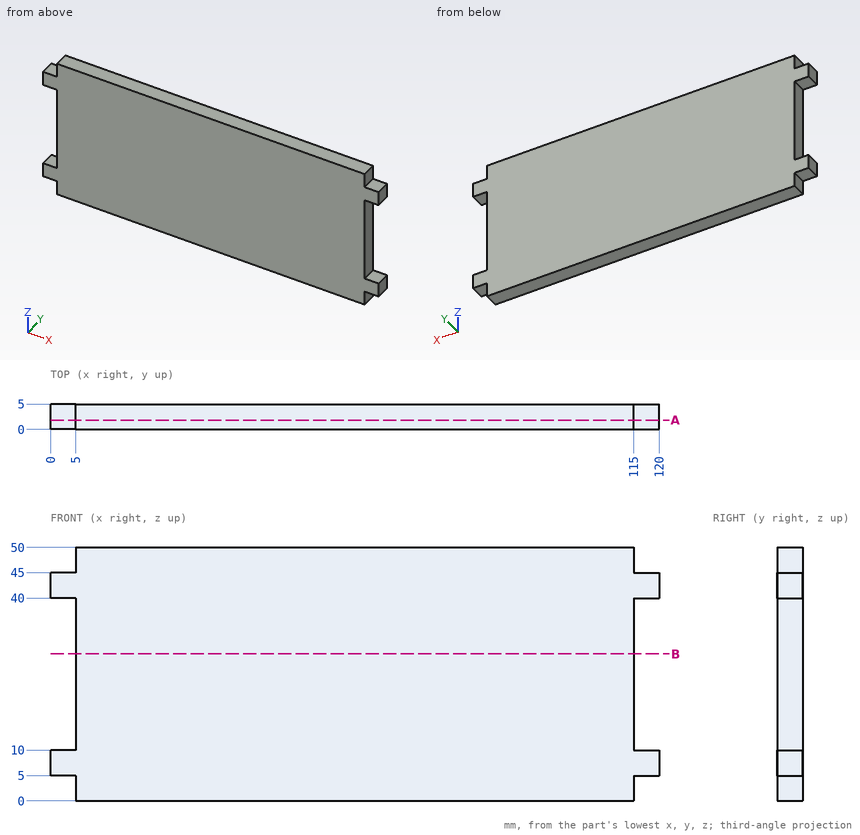
The drawing under review shows one solid part. Ordinate dimensions are in mm from its lowest x, y, z. Coordinates: 2 decimals unless noted, no trailing zeros. Loops run counter-clockwise (first coordinate to the right, second up) from the corner with the lowest first, then second, coordinate; pieces in that order, holes last.
Item 1: Clearance check with flat-ended pins moving along their axes: pin 1 (2.5 mm diameter, centred on x = 2.5, y = 3.5, fed in from -Z); pin 2 (2.5 mm diameter, centred on y = 3, z = 19.5, fed in from +X); pin 3 (2.5 mm diameter, centred on y = 1.5, z = 46.5, fed in from -X). State where each tip first meets the part, or that it passes through.
Completed:
pin 1: stops at z = 5
pin 2: stops at x = 115
pin 3: stops at x = 5
Item 2: Add section A-A (y = 1.8). Write out the cut boundary in (x, z).
Completed:
outline: (0, 5) - (5, 5) - (5, 0) - (115, 0) - (115, 5) - (120, 5) - (120, 10) - (115, 10) - (115, 40) - (120, 40) - (120, 45) - (115, 45) - (115, 50) - (5, 50) - (5, 45) - (0, 45) - (0, 40) - (5, 40) - (5, 10) - (0, 10) - close
Item 3: Add section B-B (z = 29). Write out the cut boundary in (x, y).
Completed:
outline: (5, 0) - (115, 0) - (115, 5) - (5, 5) - close
Item 4: Wall thickness on L1, parallel to X at y = 3.1, z = 12.5: over which ranges is the line inside the solid? List them lowest first.
Completed:
L1: x = 5 to 115
